The listing builds one solid part. Answer for the finished solid, in the listing's coordinates (mm). Face numbers are marked on the shaded views. A direction names the side the tool comes from. Round coordinates to 2 decimals unless told otherwise and drop trailing zeros. Write each loop counter-clockwise with the first axis right and the second up, starting at its lowest first coordinate (ties: lowest second). Pieces come first, ordered by that corner, then holes. Notation, with made-up numbers: M 66.25,58 L 100.25,58 A15 ccw 100.25,70 Z; hole C 6.25,71 d6. An arc over 180 degrees is marked long. Put each result on its own line as item: value. Start each with the question number.
```python
from build123d import *

# Parameters (mm, degrees)
SKETCH1_W               = 64.75
SKETCH1_H               = 83.69
SKETCH1_R               = 1.35
BOSS_EXTRUDE1_DEPTH     = 25.4
CUT_EXTRUDE1_DEPTH      = 82.17097095
SKETCH5_W               = 58.29
SKETCH5_H               = 20.6375
CUT_EXTRUDE3_DEPTH      = 82.17097095
BOSS_EXTRUDE2_START     = 4.7625
SKETCH1_3_W             = 6.75
SKETCH1_3_H             = 6.75
SKETCH1_3_R             = 1.35
SKETCH1_3_H_2           = 2.54
BOSS_EXTRUDE2_DEPTH     = 12.7
CUT_EXTRUDE6_DEPTH      = 55.409876401
CUT_EXTRUDE6_DEPTH_BACK = 55.409876401
SKETCH7_W               = 26.65
SKETCH7_H               = 12.7
SKETCH7_W_2             = 7.249
SKETCH7_H_2             = 55.115
SKETCH26_W              = 12.7
SKETCH26_H              = 6.35
CUT_EXTRUDE17_DEPTH     = 82.17097095
SKETCH22_W              = 17.625
SKETCH22_H              = 3.2375
BOSS_EXTRUDE6_DEPTH     = 3.175


with BuildPart() as part:
    # Sketch1 → Boss-Extrude1 (new body)
    with BuildSketch(Plane(origin=(0, 0, 0), x_dir=(1, 0, 0), z_dir=(0, 1, 0))):
        Rectangle(SKETCH1_W, SKETCH1_H)
        with Locations(Location((-29, 10.53, 0), (0, 0, 270))):
            Circle(SKETCH1_R, mode=Mode.SUBTRACT)
        with Locations(Location((-29, -38.47, 0), (0, 0, 270))):
            Circle(SKETCH1_R, mode=Mode.SUBTRACT)
        with Locations(Location((29, 10.53, 0), (0, 0, 270))):
            Circle(SKETCH1_R, mode=Mode.SUBTRACT)
        with Locations(Location((29, -38.47, 0), (0, 0, 270))):
            Circle(SKETCH1_R, mode=Mode.SUBTRACT)
    extrude(amount=BOSS_EXTRUDE1_DEPTH)

    # Sketch3 → Cut-Extrude1 (cut, through all)
    with BuildSketch(Plane(origin=(32.375, 0, 0), x_dir=(0, 0, -1), z_dir=(1, 0, 0))):
        Polygon((41.845, 18.034), (22.795, 18.669), (22.795, 12.7), (41.845, 12.7), align=None)
        Polygon((41.845, 25.4), (22.795, 25.4), (41.845, 24.765), align=None)
    extrude(amount=-CUT_EXTRUDE1_DEPTH, mode=Mode.SUBTRACT)

    # Sketch5 → Cut-Extrude3 (cut, through all)
    with BuildSketch(Plane(origin=(32.375, 0, 0), x_dir=(0, 0, -1), z_dir=(1, 0, 0))):
        with Locations((-12.7, 15.08125)):
            Rectangle(SKETCH5_W, SKETCH5_H)
    extrude(amount=-CUT_EXTRUDE3_DEPTH, mode=Mode.SUBTRACT)

    # Sketch1<3> → Boss-Extrude2 (add)
    # profile 1 of 6: a face of its own
    with BuildSketch(Plane(origin=(0, 0, 0), x_dir=(1, 0, 0), z_dir=(0, 1, 0)).offset(BOSS_EXTRUDE2_START)):
        with Locations((29, -38.47)):
            Rectangle(SKETCH1_3_W, SKETCH1_3_H)
        with Locations(Location((29, -38.47, 0), (0, 0, 90))):
            Circle(SKETCH1_3_R, mode=Mode.SUBTRACT)
    # profile 2 of 6: a face of its own
    with BuildSketch(Plane(origin=(0, 0, 0), x_dir=(1, 0, 0), z_dir=(0, 1, 0)).offset(BOSS_EXTRUDE2_START)):
        with Locations((-29, -38.47)):
            Rectangle(SKETCH1_3_W, SKETCH1_3_H)
        with Locations(Location((-29, -38.47, 0), (0, 0, 90))):
            Circle(SKETCH1_3_R, mode=Mode.SUBTRACT)
    # profile 3 of 6: a face of its own
    with BuildSketch(Plane(origin=(0, 0, 0), x_dir=(1, 0, 0), z_dir=(0, 1, 0)).offset(BOSS_EXTRUDE2_START)):
        with Locations((-29, 10.53)):
            Rectangle(SKETCH1_3_W, SKETCH1_3_H)
        with Locations(Location((-29, 10.53, 0), (0, 0, 90))):
            Circle(SKETCH1_3_R, mode=Mode.SUBTRACT)
    # profile 4 of 6: a face of its own
    with BuildSketch(Plane(origin=(0, 0, 0), x_dir=(1, 0, 0), z_dir=(0, 1, 0)).offset(BOSS_EXTRUDE2_START)):
        with Locations((29, 10.53)):
            Rectangle(SKETCH1_3_W, SKETCH1_3_H)
        with Locations(Location((29, 10.53, 0), (0, 0, 90))):
            Circle(SKETCH1_3_R, mode=Mode.SUBTRACT)
    # profile 5 of 6: a face of its own
    with BuildSketch(Plane(origin=(0, 0, 0), x_dir=(1, 0, 0), z_dir=(0, 1, 0)).offset(BOSS_EXTRUDE2_START)):
        with Locations((-29, 15.175)):
            Rectangle(SKETCH1_3_W, SKETCH1_3_H_2)
    # profile 6 of 6: a face of its own
    with BuildSketch(Plane(origin=(0, 0, 0), x_dir=(1, 0, 0), z_dir=(0, 1, 0)).offset(BOSS_EXTRUDE2_START)):
        with Locations((29, 15.175)):
            Rectangle(SKETCH1_3_W, SKETCH1_3_H_2)
    extrude(amount=BOSS_EXTRUDE2_DEPTH)

    # Sketch7 → Cut-Extrude6 (cut, two sides: drawn at the far end of the back side and taken through both)
    with BuildSketch(Plane(origin=(0, 12.7, 0), x_dir=(1, 0, 0), z_dir=(0, 1, 0)).offset(-CUT_EXTRUDE6_DEPTH_BACK)):
        Polygon((-13.325, 16.445), (-13.325, -38.67), (13.325, -38.67), (13.325, 16.445), (13.325, 22.795), (-13.325, 22.795), align=None)
        with Locations((0, 29.145)):
            Rectangle(SKETCH7_W, SKETCH7_H)
        with Locations((-16.9495, -11.1125)):
            Rectangle(SKETCH7_W_2, SKETCH7_H_2)
        with Locations((16.9495, -11.1125)):
            Rectangle(SKETCH7_W_2, SKETCH7_H_2)
    extrude(amount=CUT_EXTRUDE6_DEPTH + CUT_EXTRUDE6_DEPTH_BACK, mode=Mode.SUBTRACT)

    # Sketch26 → Cut-Extrude17 (cut, through all)
    with BuildSketch(Plane(origin=(32.375, 0, 0), x_dir=(0, 0, -1), z_dir=(1, 0, 0))):
        with Locations((29.145, 3.175)):
            Rectangle(SKETCH26_W, SKETCH26_H)
    extrude(amount=-CUT_EXTRUDE17_DEPTH, mode=Mode.SUBTRACT)

    # Fillet1
    # an asymmetric fillet: 3.175, 1.905 mm, written as the material it takes off along each edge
    with BuildSketch(Plane(origin=(40.475658498, 18.034, -41.845), x_dir=(0, 1, 0), z_dir=(-1, 0, 0))) as fillet1_piece_1:
        with BuildLine():
            Bezier((2.011891373, 0), (0, 0), (0.107948825, -3.238464752), weights=[1, 0.695228441, 1])
            Line((0.107948825, -3.238464752), (0, 0))
            Line((0, 0), (2.011891373, 0))
        make_face()
    extrude(amount=80.951316996, mode=Mode.SUBTRACT)

    # Sketch22 → Boss-Extrude6 (add)
    with BuildSketch(Plane.XY.offset(41.845)):
        with Locations((-16.8125, 6.38125)):
            Rectangle(SKETCH22_W, SKETCH22_H)
        with Locations((16.8125, 6.38125)):
            Rectangle(SKETCH22_W, SKETCH22_H)
    extrude(amount=-BOSS_EXTRUDE6_DEPTH)


solid = part.part
```
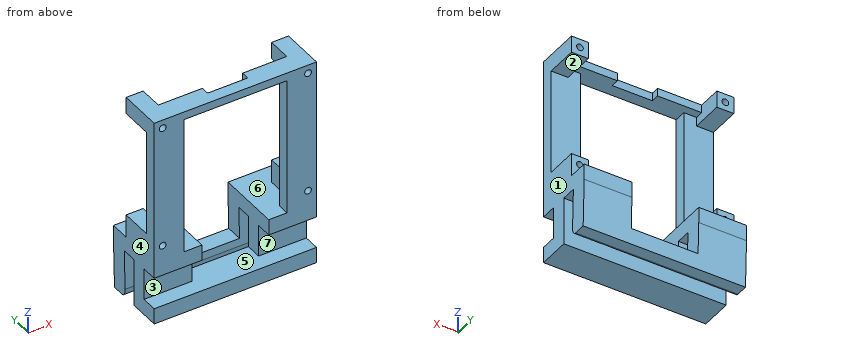
Item 1: Section A-A (y = 9) is taken. Give the vertices of the cut face in (x, z) (3 decimals), and give its area (3 significant figures).
Item 2: Section B-B (z = -10.53) is taken. Count the separate pieces of the cut face and the enclosed holes in it, and give its area (3 significant figures).
Item 3: Consider line 1 along Z through (x, y) = (29, 11.5) (3 decimals); line 2 along X through (y, z) = (10.5, 38.47) (3 decimals); line 3 along Z through (x, y) = (-29, 4.5) (3 decimals). Determine where each line is inside the solid, lowest interval first. Write a range as [from, to].
Item 4: Determine the mould class of the marked faces 4, 5, 6 and 7 for opening direction X: released by +X, released by -X, zero draft, split by the parting line, or undercut.
Item 5: Flat-ended cylindrical pins translate along their axes: pin 1 (5 mm diameter, centred on x = 21, y = 11, fed in from +Z) (3 decimals); pin 2 (3.5 mm diameter, centred on x = -29, z = 38.47, fed in from +Y); pin 3 (15 mm diameter, centred on x = 12.5, z = -35, fed in from +Y). Find the tip coordinate at first contact, or state that the pin passes through.
Item 6: Section C-C (z = 30) is taken. Give the vertices of the cut face in (x, y) (1 decimal).
Item 7: Which of the six approach directions +Z, -Z, +X, -X, +Y, -Y give full straight-line access (tool end or side, diameter ignored) to the marked faces 1, 2 and 3?
Output values:
1. outline: M -32.375,-41.845 L 32.375,-41.845 L 32.375,-7.155 L 25.625,-7.155 L 25.625,-16.445 L 13.325,-16.445 L 13.325,-35.495 L -13.325,-35.495 L -13.325,-16.445 L -25.625,-16.445 L -25.625,-7.155 L -32.375,-7.155 Z; M -32.375,35.095 L -25.625,35.095 L -25.625,41.845 L -32.375,41.845 Z; M 25.625,35.095 L 32.375,35.095 L 32.375,41.845 L 25.625,41.845 Z; hole C -29,-10.53 d2.7; hole C -29,38.47 d2.7; hole C 29,-10.53 d2.7; hole C 29,38.47 d2.7
1. area: 1,330 mm^2
2. separate pieces: 4
2. enclosed holes: 0
2. area: 190 mm^2
3. line 1: z = [-41.845, -11.88], [-9.18, -7.155], [35.095, 37.12], [39.82, 41.845]
3. line 2: x = [-32.375, -30.35], [-27.65, -25.625], [25.625, 27.65], [30.35, 32.375]
3. line 3: z = [-41.845, -35.495], [-22.795, -11.88], [-9.18, 37.12], [39.82, 41.845]
4. face 4: released by -X
4. face 5: undercut
4. face 6: undercut
4. face 7: zero draft
5. pin 1: stops at z = -16.445
5. pin 2: stops at y = 17.46
5. pin 3: stops at y = 25.24
6. outline: M -32.4,0 L -20.6,0 L -20.6,4.8 L -32.4,4.8 Z; M 20.6,0 L 32.4,0 L 32.4,4.8 L 20.6,4.8 Z
7. face 1: +Z, -Z, +X, +Y, -Y
7. face 2: +X, -X, +Y
7. face 3: +X, -X, -Y
